from build123d import *

# Parameters (mm, degrees)
SKETCH1_W           = 700
SKETCH1_H           = 350
BOSS_EXTRUDE1_DEPTH = 2.54
SKETCH2_W           = 10
SKETCH2_H           = 350
SKETCH2_H_2         = 330
BOSS_EXTRUDE2_DEPTH = 0.254
SCALE1_SCALE        = 1.5


with BuildPart() as part:
    # Sketch1 → Boss-Extrude1 (new body)
    with BuildSketch(Plane(origin=(0, 0, 0), x_dir=(1, 0, 0), z_dir=(0, 1, 0))):
        Rectangle(SKETCH1_W, SKETCH1_H)
    extrude(amount=BOSS_EXTRUDE1_DEPTH)

    # Sketch2 → Boss-Extrude2 (add)
    with BuildSketch(Plane(origin=(0, 2.54, 0), x_dir=(1, 0, 0), z_dir=(0, 1, 0))):
        Polygon((-316.560265613, 175), (-350, 175), (-333.280132806, 48), align=None)
        Polygon((-272.110265613, 175), (-305.55, 175), (-288.830132806, 48), align=None)
        Polygon((-227.660265613, 175), (-261.1, 175), (-244.380132806, 48), align=None)
        Polygon((-183.210265613, 175), (-216.65, 175), (-199.930132806, 48), align=None)
        Polygon((-138.760265613, 175), (-172.2, 175), (-155.480132806, 48), align=None)
        Polygon((-94.310265613, 175), (-127.75, 175), (-111.030132806, 48), align=None)
        with Locations((-72.168132806, 0)):
            Rectangle(SKETCH2_W, SKETCH2_H)
        Polygon((-16.586265613, 175), (-50.026, 175), (-33.306132806, 48), align=None)
        Polygon((27.863734387, 175), (-5.576, 175), (11.143867194, 48), align=None)
        Polygon((72.313734387, 175), (38.874, 175), (55.593867194, 48), align=None)
        Polygon((116.763734387, 175), (83.324, 175), (100.043867194, 48), align=None)
        Polygon((161.213734387, 175), (127.774, 175), (144.493867194, 48), align=None)
        Polygon((205.663734387, 175), (172.224, 175), (188.943867194, 48), align=None)
        Polygon((-350, -175), (-316.560265613, -175), (-333.280132806, -48), align=None)
        Polygon((-305.55, -175), (-272.110265613, -175), (-288.830132806, -48), align=None)
        Polygon((-261.1, -175), (-227.660265613, -175), (-244.380132806, -48), align=None)
        Polygon((-216.65, -175), (-183.210265613, -175), (-199.930132806, -48), align=None)
        Polygon((-172.2, -175), (-138.760265613, -175), (-155.480132806, -48), align=None)
        Polygon((-127.75, -175), (-94.310265613, -175), (-111.030132806, -48), align=None)
        Polygon((-33.306132806, -48), (-50.026, -175), (-16.586265613, -175), align=None)
        Polygon((11.143867194, -48), (-5.576, -175), (27.863734387, -175), align=None)
        Polygon((55.593867194, -48), (38.874, -175), (72.313734387, -175), align=None)
        Polygon((100.043867194, -48), (83.324, -175), (116.763734387, -175), align=None)
        Polygon((144.493867194, -48), (127.774, -175), (161.213734387, -175), align=None)
        Polygon((188.943867194, -48), (172.224, -175), (205.663734387, -175), align=None)
        Polygon((241.063734387, 175), (231.063734387, 175), (231.063734387, -175), (241.063734387, -175), (241.063734387, -165), (241.063734387, 165), align=None)
        Polygon((241.063734387, -165), (241.063734387, -175), (350, -175), (350, -165), (340, -165), align=None)
        with Locations((345, 0)):
            Rectangle(SKETCH2_W, SKETCH2_H_2)
        Polygon((350, 175), (241.063734387, 175), (241.063734387, 165), (340, 165), (350, 165), align=None)
    extrude(amount=BOSS_EXTRUDE2_DEPTH)


with BuildPart() as part_1:
    # Scale1: scaled about (-0.525903048, 1.305261187, 0)
    add(part.part.scale(SCALE1_SCALE).moved(Location((0.262951524, -0.652630593, 0))))


solid = part_1.part
The model under review builds one solid part; all positions refer to its coordinate system, in mm. A direction names the side the tool comes from. Round coordinates to 2 decimals unless told otherwise and drop trailing zeros. Order: outer loops, then holes, each group sorted by start corner. A loop starts at its lowest first (then second) coordinate and runs counter-clockwise, first axis right, second up. Notation, with made-up numbers: (57, 67.5) -> (104, 67.5) arc R15 ccw to (104, 90.5) -> close; hole circle Ø5 at (15.5, 43). An arc over 180 degrees is marked (long way). Write item = value, one per line. Start each with the question number.
Item 1: Consider section B-B on x = 97.5. Write out the cut boundary in (y, z).
Item 2: Consider section A-A on z = -46. Write out the cut boundary in (x, y), plus the area to 3 significant figures.
Item 3: Mouldability with a two-part tool opening along Z and no side actions: class faces 1 (the face through (162.693, 3.345, -165.916)), 2 (the face through (283, 3.538, -190)) as released by +Z, released by -Z, zero draft, split by the parting line, or undercut.
Item 4: For faces 3 (the face through (217, 3.538, -190)), 4 (the face through (4.614, 3.345, 165.916)), list the 3-axis set-ups (+Z, -Z, +X, -X, +Y, -Y) from which the entire face can be reached by the end or side of a thin tool; tool diameter is ignored.
Item 5: Consider section C-C on x = 403. Write out the cut boundary in (y, z), plus the area to 3 significant figures.
Item 6: For line 1 along Y through (x, z) = (236.5, 19.5), list the stretches that pass through material, from the lowest coordinate up.
Conclusion:
q1.outline = (-0.65, -262.5) -> (3.54, -262.5) -> (3.54, -177.17) -> (3.16, -177.17) -> (3.16, 177.17) -> (3.54, 177.17) -> (3.54, 262.5) -> (-0.65, 262.5) -> close
q2.outline = (-524.74, -0.65) -> (525.26, -0.65) -> (525.26, 3.54) -> (510.26, 3.54) -> (510.26, 3.16) -> (361.86, 3.16) -> (361.86, 3.54) -> (346.86, 3.54) -> (346.86, 3.16) -> (-100.49, 3.16) -> (-100.49, 3.54) -> (-115.49, 3.54) -> (-115.49, 3.16) -> (-524.74, 3.16) -> close
q2.area = 4,020 mm2
q3.face_1 = undercut
q3.face_2 = zero draft
q4.face_3 = +Z, -Z, +X, -X, +Y
q4.face_4 = +Y
q5.outline = (-0.65, -262.5) -> (3.54, -262.5) -> (3.54, -247.5) -> (3.16, -247.5) -> (3.16, 247.5) -> (3.54, 247.5) -> (3.54, 262.5) -> (-0.65, 262.5) -> close
q5.area = 2,010 mm2
q6.line_1 = -0.65 to 3.16
